Part model, mm, in its own coordinate system. Give positions to 0.01 mm unless a question says otherwise; leave off trailing zeros. Write each loop counter-clockwise with the first axis right and the second up, starting at its lowest first coordinate (ties: lowest second). Pieces come first, ordered by that corner, then holes. Notation, with made-up numbers: (22, 32.25) - (51, 32.25) arc R4 cw to (51, 38.25) - close; hole circle Ø3 at (36.5, -25). An arc over 180 degrees is marked (long way). Answer in a Markdown table with one row per item. Add a question column.
1. Probe line 1 along X through (y, z) = (3.05, -23.5); line 2 along X through (y, z) = (5, -22.5); line 3 along Z through (x, y) = (35.5, 1.1). List the from-to ranges inside material, lowest first.
2. Pull direction Z, two halves, no side cores. Call faces 1 (the cylindrical face through (35.783, 3.042, -10.767)), 2 (the flat face through (25, 3, 0)), 3 (the cylindrical face through (49.4, 5.43, -14.96)), 4 (the cylindrical face through (35.783, 3.042, -23.767)): released by +Z, released by -Z, zero draft, split by the parting line, or undercut.
3. Band-saw the part on C-C on x = 16.25. Write the cut outline in (y, z), plus the area to 3 significant figures.
4. Band-saw the part on D-D on y = 4.6. Write the cut outline in (x, z).
5. Band-saw the part on A-A on z = -23.5. Write the cut outline in (x, y).
6. Drop a flat-ended pin along its axis: pin 1 Ø3.5 at (x, z) = (16.25, -10.5) entering from -Y. Give the stop position or say it passes through.
7. Band-saw the part on B-B on y = 1.25. Write the cut outline in (x, z), plus the area to 3 significant figures.
```python
from build123d import *

# Parameters (mm, degrees)
SKETCH1_W             = 17.5
SKETCH1_H             = 6
SKETCH1_H_2           = 13
SKETCH1_W_2           = 16.25
SKETCH1_H_3           = 10.5
BOSS_EXTRUDE1_DEPTH   = 6
FILLET1_R             = 2
FILLET2_R             = 2
F_4_0MM_DOWEL_HOLE2_D = 4.1


with BuildPart() as part:
    # Sketch1 → Boss-Extrude1 (new body)
    with BuildSketch(Plane(origin=(0, 0, 0), x_dir=(1, 0, 0), z_dir=(0, 1, 0))):
        Polygon((0, 0), (16.25, 0), (16.25, 10.5), (16.25, 23.5), (16.25, 29.5), (0, 29.5), align=None)
        with Locations((25, 26.5)):
            Rectangle(SKETCH1_W, SKETCH1_H)
        with Locations((25, 17)):
            Rectangle(SKETCH1_W, SKETCH1_H_2)
        with Locations((41.875, 17)):
            Rectangle(SKETCH1_W_2, SKETCH1_H_2)
        with Locations((25, 5.25)):
            Rectangle(SKETCH1_W, SKETCH1_H_3)
        with Locations((41.875, 5.25)):
            Rectangle(SKETCH1_W_2, SKETCH1_H_3)
        with Locations((41.875, 26.5)):
            Rectangle(SKETCH1_W_2, SKETCH1_H)
    extrude(amount=BOSS_EXTRUDE1_DEPTH)

    # Fillet1
    fillet1_edges = [part.edges().sort_by_distance(p)[0] for p in [
        (0, 6, -14.75),
    ]]
    fillet(fillet1_edges, radius=FILLET1_R)

    # Fillet2
    fillet2_edges = [part.edges().sort_by_distance(p)[0] for p in [
        (50, 6, -14.75),
    ]]
    fillet(fillet2_edges, radius=FILLET2_R)

    # Ø4.0mm Dowel Hole2 (through all)
    with Locations(Plane(origin=(16.25, 0, -23.5), x_dir=(0, 0, -1), z_dir=(0, -1, 0))):
        with Locations((0, 0), (0, 17.5), (-13, 17.5), (-13, 0)):
            Hole(F_4_0MM_DOWEL_HOLE2_D / 2)


solid = part.part
```
Values:
| question | item | result |
|---|---|---|
| 1 | line 1 | x = 0 to 14.2, 18.3 to 31.7, 35.8 to 50 |
| 1 | line 2 | x = 0.27 to 14.46, 18.04 to 31.96, 35.54 to 49.73 |
| 1 | line 3 | z = -29.5 to -24.57, -22.43 to -11.57, -9.43 to 0 |
| 2 | face 1 | undercut |
| 2 | face 2 | released by +Z |
| 2 | face 3 | zero draft |
| 2 | face 4 | undercut |
| 3 | outline | (0, -29.5) - (6, -29.5) - (6, -25.55) - (0, -25.55) - close; (0, -21.45) - (6, -21.45) - (6, -12.55) - (0, -12.55) - close; (0, -8.45) - (6, -8.45) - (6, 0) - (0, 0) - close |
| 3 | area | 128 mm² |
| 4 | outline | (0.09, -29.5) - (49.91, -29.5) - (49.91, 0) - (0.09, 0) - close; hole circle Ø4.1 at (16.25, -23.5); hole circle Ø4.1 at (16.25, -10.5); hole circle Ø4.1 at (33.75, -23.5); hole circle Ø4.1 at (33.75, -10.5) |
| 5 | outline | (0, 0) - (14.2, 0) - (14.2, 6) - (2, 6) arc R2 ccw to (0, 4) - close; (18.3, 0) - (31.7, 0) - (31.7, 6) - (18.3, 6) - close; (35.8, 0) - (50, 0) - (50, 4) arc R2 ccw to (48, 6) - (35.8, 6) - close |
| 6 | pin 1 | passes through |
| 7 | outline | (0, -29.5) - (50, -29.5) - (50, 0) - (0, 0) - close; hole circle Ø4.1 at (16.25, -23.5); hole circle Ø4.1 at (16.25, -10.5); hole circle Ø4.1 at (33.75, -23.5); hole circle Ø4.1 at (33.75, -10.5) |
| 7 | area | 1,420 mm² |
